Can you work these out from the model? Positions are in its coordinate system, mm. A direction names the side the tool comes from. Round coordinates to 2 decimals unless told otherwise and drop trailing zeros. Loops run counter-clockwise (first coordinate to the right, second up) from the corner with the lowest first, then second, coordinate; pieces in that order, holes last.
(1) If I drill on line 1 along X through (y, z) = (0.2, -1.15); line 2 along Z through (x, y) = (0.5, -0.65); line 3 along X through (y, z) = (-1.2, -1.2), over which ranges is the centre line in solid material (lowest first)?
(2) I want a section at A-A on x = 7. Write out the boundary of the cut face in (y, z).
(3) Will this pin go through, and if not, where does the flat tip stop? pin 1 Ø1 at (y, z) = (1, 1) entering from -X.
(4) Thinking about a two-plate mould opening in Y: for faces 4 (the face through (5.09, -0.27, 1.22)), 5 (the face through (0.474, 0.253, 0.82)), 6 (the face through (8, 0, 0)), which applies, released by +Y, released by -Y, zero draft, split by the parting line, or undercut?
(5) Which directions (+Z, -Z, +X, -X, +Y, -Y) give clear straight access to the entire face, cutting with the end or side of a thin tool? Please do faces 1 (the face through (0, 0.5, -0.5)), 2 (the face through (0.474, -0.253, 0.82)), 3 (the face through (1.81, 1.06, -0.33)).
Autodesk Inventor part; units mm, degrees
ref_plane "Work Plane2" through (3.35, 0, 0) normal (0, 0, -1) x (1, 0, 0)
ref_plane "YZ Plane" through (0, 0, 0) normal (1, 0, 0) x (0, 1, 0)
ref_plane "XZ Plane" through (0, 0, 0) normal (0, 1, 0) x (-1, 0, 0)
sketch "Szkic1" plane through (0, 0, 0) normal (0, 0, 1) x (1, 0, 0)
  line L0 (1.48, 0) -> (8, 0)
  line L1 (8, 0) -> (8, 1.25)
  line L2 (8, 1.25) -> (2.4, 1.25)
  line L3 (2.4, 1.25) -> (2.1239, 1.112)
  line L4 (2.1239, 1.112) -> (1.5, 1.112)
  line L5 (0, 2.2) -> (0, 1.385)
  line L6 (0, 1.385) -> (1.0118, 0.8805)
  line L7 (1.0118, 0.8805) -> (1.48, 0)
  line L8 (-1.6, 0) -> (9.6, 0)
  line L9 (0, -0.44) -> (0, 2.64)
  line L10 (0, 2.2) -> (0.412, 2.2)
  line L11 (0.412, 2.2) -> (1.5, 1.112)
  line L12 (2.4, 1.25) -> (1.362, 1.25) construction
  dimension "d1" = 5.6
  dimension "d2" = 2.5
  dimension "d3" = 2.2239
  dimension "d4" = 2.77
  dimension "d5" = 26.5
  dimension "d6" = 62
  dimension "d7" = 1.48
  dimension "d8" = 0.2761
  dimension "d12" = 4.4
  dimension "d13" = 45
  dimension "d15" = 8
  dimension "d24" = 1.5
revolve "Bryła" add sketch "Szkic1" angle 360 about axis through (1.48, 0, 0) along (1, 0, 0) contours L7 L6 L5 L10 L11 L4 L3 L2 L1 L0
sketch "Szkic2" plane through (0, 0, 0) normal (-1, 0, 0) x (0, 0, 1)
  line L0 (0, 1.385) -> (0, 0) construction
  line L1 (0, 0) -> (1.385, 0) construction
  arc A0 (0.4155, 0) -> (0, 0.4155) centre (0, 0) ccw construction
  arc A1 (0.4848, 0) -> (0, 0.4848) centre (0, 0) ccw construction
  arc A2 (1.34, 0.35) -> (0.35, 1.34) centre (0, 0) ccw
  line L2 (0, 0) -> (0.9793, 0.9793) construction
  line L3 (0.35, 1.34) -> (0.2511, 0.4146)
  line L4 (1.34, 0.35) -> (0.4146, 0.2511)
  arc A3 (0.35, 1.34) -> (0, 1.385) centre (0, 0) ccw
  arc A4 (1.385, 0) -> (1.34, 0.35) centre (0, 0) ccw
  line L5 (0, -3.08) -> (0, 3.08)
  line L6 (-3.08, 0) -> (3.08, 0)
  arc A5 (0.35, -1.34) -> (1.34, -0.35) centre (0, 0) ccw
  line L7 (0.35, -1.34) -> (0.2511, -0.4146)
  line L8 (1.34, -0.35) -> (0.4146, -0.2511)
  arc A6 (0, -1.385) -> (0.35, -1.34) centre (0, 0) ccw
  arc A7 (1.34, -0.35) -> (1.385, 0) centre (0, 0) ccw
  arc A8 (-0.35, 1.34) -> (-1.34, 0.35) centre (0, 0) ccw
  line L9 (-0.35, 1.34) -> (-0.2511, 0.4146)
  line L10 (-1.34, 0.35) -> (-0.4146, 0.2511)
  arc A9 (0, 1.385) -> (-0.35, 1.34) centre (0, 0) ccw
  arc A10 (-1.34, 0.35) -> (-1.385, 0) centre (0, 0) ccw
  arc A11 (-0.35, -1.34) -> (0, -1.385) centre (0, 0) ccw
  arc A12 (-1.34, -0.35) -> (-0.35, -1.34) centre (0, 0) ccw
  arc A13 (-1.385, 0) -> (-1.34, -0.35) centre (0, 0) ccw
  line L11 (-1.34, -0.35) -> (-0.4146, -0.2511)
  line L12 (-0.35, -1.34) -> (-0.2511, -0.4146)
  arc A14 (0.2511, 0.4146) -> (0.4146, 0.2511) centre (0.3988, 0.3988) ccw
  arc A15 (0.4146, -0.2511) -> (0.2511, -0.4146) centre (0.3988, -0.3988) ccw
  arc A16 (-0.4146, 0.2511) -> (-0.2511, 0.4146) centre (-0.3988, 0.3988) ccw
  arc A17 (-0.2511, -0.4146) -> (-0.4146, -0.2511) centre (-0.3988, -0.3988) ccw
  point P0 (0.9793, -0.9793)
  point P1 (-0.9793, 0.9793)
  point P2 (-0.9793, -0.9793)
  dimension "d17" = 0.831
  dimension "d18" = 0.9695
  dimension "d19" = 2.77
  dimension "d20" = 45
  dimension "d21" = 0.35
extrude "Szczelina" add sketch "Szkic2" against normal up to next draft 5 contours L4 A14 L3 A2 | A5 L7 A15 L8 | L9 A16 L10 A8 | A12 L11 A17 L12
fillet "Zaokrąglenie1" radius 0.14 4 edges at (0, 1.385, 0) (0, 0, -1.385) (0, -1.385, 0) (0, 0, 1.385)
thread "Gwint"
chamfer "Faza1" distance 0.2761 distance2 0.138 1 edges at (8, -1.25, 0) measured on face at (8, -0.3689, 0.1936)
ref_plane "Work Plane2" through (3.35, 0, 0) normal (0, 0, -1) x (1, 0, 0)
equation "\"d1\" = GEL"
equation "\"d2\" = GD"
equation "\"d3\" = BDM"
equation "\"d4\" = SDM"
equation "\"d7\" = INTI"
equation "\"d8\" = GAL"
equation "\"d12\" = KOD"
equation "\"d13\" = 0.5 * SEWI"
equation "\"d15\" = NLG"
equation "\"d24\" = KOH"
equation "\"d17\" = 0.3 * SDM"
equation "\"d18\" = 0.35 * SDM"
equation "\"d19\" = SDM"
equation "\"d21\" = 0.5 * SBR"
equation "\"d23\" = 0.2 * SBR"
equation "\"d10\" = GEL"
equation "\"d25\" = -0.5 * SPD + 0.5 * GD"
equation "\"d26\" = 0.5 * GAL"
equation "\"NLG\" = 8"
equation "\"GEL\" = 5.6"
equation "\"GAL\" = 0.61345 * PTC"
equation "\"SPD\" = NND - 1.2269 * PTC"
equation "\"KOD\" = 4.4"
equation "\"KOH\" = 1.5"
equation "\"SBR\" = 0.7"
equation "\"INTI\" = 1.48"
equation "\"SDM\" = 2.77"
equation "\"GD\" = NND"
equation "\"BDM\" = NND - GAL"
equation "\"SEWI\" = 90deg"
equation "\"d9\" = SDM"
equation "\"GUL\" = 0.61345 * PTC"
equation "\"TOA\" = 30deg"
equation "\"EPV\" = 2.75"
equation "\"THREADDIA\" = 2.5"
equation "\"RR\" = 0.3"
equation "\"PTC\" = 0.45"
equation "\"NND\" = 2.5"
equation "\"GD1\" = THREADDIA - 1.2269 * PTC"
properties part number "AS 1427 - M2,5 x 8" material "Stal, miękka"
Filled sheet:
1. line 1: x = 0.44 to 1.44, 2.23 to 7.9
1. line 2: z = -2.01 to -0.23, 0.23 to 2.01
1. line 3: x = 0 to 0.91
2. outline: circle Ø2.5 at (0, 0)
3. pin 1: stops at x = 0
4. face 4: split by the parting line
4. face 5: undercut
4. face 6: zero draft
5. face 1: +Z, -Z, -X, +Y, -Y
5. face 2: -X
5. face 3: none
